Source: CAD feature listing. Evaluate the final solid. Frame: model axes, mm. A direction names the side the tool comes from. Round coordinates to 2 decimals unless told otherwise and drop trailing zeros. Loops run counter-clockwise (first coordinate to the right, second up) from the corner with the lowest first, then second, coordinate; pieces in that order, holes last.
(1) Section D-D, the plane y = 2.5. Return the cut outline in (x, z).
(2) Mould query, pull axis Y, two halves, no side actions, for faces 1 (the cylindrical face through (0.65, 3.51, 0.06)), 2 (the cylindrical face through (-0.16, 78.69, 0.06)), 3 (the cylindrical face through (-1.08, 64.46, -4.88)), 4 (the flat face through (4, 13, -2)). Classes: pulls with the +Y half, pulls with the -Y half, needs draft (parallel to the pull), parting line crosses it, or undercut.
(3) Material intervals for probe 1 along Y at (x, z) = (0, -0.5); probe 2 along Y at (x, z) = (0.5, 0.5); probe 3 along X at (y, z) = (47, 0.25), sorted ascending.
(4) Section A-A, the plane x = 0. Count the separate pieces of the cut face and the enclosed holes in it, plus the area to 3 significant figures.
(5) Set-up query: faces 5 (the flat face through (4, 67, -2)), 6 (the cylindrical face through (-1.823, 6.916, 3.504)), 7 (the flat face through (0, 80, 0)). Return all of +Z, -Z, +X, -X, +Y, -Y with unobstructed straight access to the full face (end or side cutting, diameter ignored); none if empty.
(6) Section C-C, the plane y = 16. Return the cut outline in (x, z).
(7) Section B-B, the plane z = 0. Return the cut outline in (x, y), plus the area to 3 significant figures.
(8) First-contact query: pin 1 Ø3 at (x, y) = (1.5, 70.5) entering from -Z; pin 2 Ø1 at (x, y) = (4, 61) entering from +Z; pin 3 Ø6 at (x, y) = (4, 27.5) entering from +Z; pin 4 Ø1.4 at (x, y) = (0, 77.5) entering from -Z. Flat tips, straight axial feed; report the tip coordinate or a pass-through.
Autodesk Inventor part; units mm, degrees
ref_plane "YZ Plane" through (0, 0, 0) normal (1, 0, 0) x (0, 1, 0)
ref_plane "XZ Plane" through (0, 0, 0) normal (0, 1, 0) x (-1, 0, 0)
ref_plane "XY Plane" through (0, 0, 0) normal (0, 0, 1) x (1, 0, 0)
sketch "Sketch1" plane through (0, 0, 0) normal (0, 1, 0) x (-1, 0, 0)
  circle A0 centre (0, 0) radius 3.95
  dimension "d0" = 7.9
extrude "Extrusion1" add sketch "Sketch1" along normal blind 13
sketch "Sketch2" plane through (0, 13, 0) normal (0, 1, 0) x (1, 0, 0)
  circle A0 centre (0, 0) radius 5
  dimension "d3" = 10
extrude "Extrusion2" add sketch "Sketch2" along normal blind 5
sketch "Sketch3" plane through (0, 18, 0) normal (0, 1, 0) x (1, 0, 0)
  circle A0 centre (0, 0) radius 6
  dimension "d6" = 12
extrude "Extrusion3" add sketch "Sketch3" along normal blind 44
sketch "Sketch4" plane through (0, 62, 0) normal (0, 1, 0) x (1, 0, 0)
  circle A0 centre (0, 0) radius 5
  dimension "d9" = 10
extrude "Extrusion4" add sketch "Sketch4" along normal blind 5
sketch "Sketch5" plane through (0, 67, 0) normal (0, 1, 0) x (1, 0, 0)
  circle A0 centre (0, 0) radius 3.95
  dimension "d12" = 7.9
extrude "Extrusion5" add sketch "Sketch5" along normal blind 13
sketch "Sketch6" plane through (0, 0, 0) normal (0, 0, 1) x (1, 0, 0)
  circle A0 centre (0, 2.5) radius 1.2
  line L0 (3.95, 0) -> (-3.95, 0)
  point P0 (0, 0)
  dimension "d15" = 2.4
  dimension "d16" = 2.5
extrude "Extrusion6" cut sketch "Sketch6" against normal through all both and the other way through all
chamfer "Chamfer1" distance 1 angle 45 1 edges at (3.95, 0, 0)
sketch "Sketch7" plane through (0, 0, 0) normal (1, 0, 0) x (0, 1, 0)
  point P0 (0, 0)
sketch "Sketch8" plane through (0, 0, 0) normal (0, 1, 0) x (-1, 0, 0)
  point P0 (0, 0)
sketch "Sketch9" plane through (0, 0, 0) normal (0, 0, 1) x (1, 0, 0)
  circle A0 centre (0, 77.5) radius 1.2
  line L0 (3.95, 80) -> (-3.95, 80)
  point P0 (0, 0)
  dimension "d22" = 2.4
  dimension "d23" = 2.5
extrude "Extrusion7" cut sketch "Sketch9" against normal through all both and the other way through all
chamfer "Chamfer2" distance 1 angle 45 1 edges at (-3.95, 80, 0)
properties part number "Wheel_axle" material "Steel, High Strength, Low Alloy"
Output values:
1. outline: (-1.2, -3.76) - (-1.2, 3.76) arc R3.95 ccw to start; (1.2, -3.76) arc R3.95 ccw to (1.2, 3.76) - close
2. face 1: undercut
2. face 2: undercut
2. face 3: needs draft
2. face 4: pulls with the -Y half
3. probe 1: y = 0 to 1.3, 3.7 to 76.3, 78.7 to 80
3. probe 2: y = 0 to 1.41, 3.59 to 76.41, 78.59 to 80
3. probe 3: x = -5.99 to 5.99
4. separate pieces: 3
4. enclosed holes: 0
4. area: 793 mm2
5. face 5: +Y
5. face 6: -Y
5. face 7: +Z, -Z, +X, -X, +Y
6. outline: circle Ø10 at (0, 0)
7. outline: (-6, 18) - (-5, 18) - (-5, 13) - (-3.95, 13) - (-3.95, 1) - (-2.95, 0) - (2.95, 0) - (3.95, 1) - (3.95, 13) - (5, 13) - (5, 18) - (6, 18) - (6, 62) - (5, 62) - (5, 67) - (3.95, 67) - (3.95, 79) - (2.95, 80) - (-2.95, 80) - (-3.95, 79) - (-3.95, 67) - (-5, 67) - (-5, 62) - (-6, 62) - close; hole circle Ø2.4 at (0, 2.5); hole circle Ø2.4 at (0, 77.5)
7. area: 822 mm2
8. pin 1: stops at z = -3.95
8. pin 2: stops at z = 4.87
8. pin 3: stops at z = 5.92
8. pin 4: passes through
